Check sheet for the modelled part. Datum: model origin and axes. Units: mm. Round coordinates to 2 decimals unless told otherwise and drop trailing zeros. Write each loop counter-clockwise with the first axis right and the second up, starting at its lowest first coordinate (ties: lowest second). Pieces come first, ordered by that corner, then holes.
from build123d import *

# Parameters (mm, degrees)
SKETCH1_W                = 132
SKETCH1_H                = 150
BOSS_EXTRUDE1_DEPTH      = 5
M6_CLEARANCE_HOLE1_D     = 6.6
M6_CLEARANCE_HOLE1_DEPTH = 10
M6_CLEARANCE_HOLE1_TIP   = 1.982840043
FILLET1_R                = 5


with BuildPart() as part:
    # Sketch1 → Boss-Extrude1 (new body)
    with BuildSketch(Plane(origin=(0, 0, 0), x_dir=(1, 0, 0), z_dir=(0, 1, 0))):
        with Locations((66, 75)):
            Rectangle(SKETCH1_W, SKETCH1_H)
    extrude(amount=BOSS_EXTRUDE1_DEPTH)

    # M6 Clearance Hole1
    with Locations(Plane(origin=(0, 0, 0), x_dir=(-1, 0, 0), z_dir=(0, -1, 0))):
        with Locations((-15, 15), (-117, 15), (-117, 135), (-15, 135)):
            Hole(M6_CLEARANCE_HOLE1_D / 2, depth=M6_CLEARANCE_HOLE1_DEPTH)
            with Locations((0, 0, -(M6_CLEARANCE_HOLE1_DEPTH + M6_CLEARANCE_HOLE1_TIP / 2))):  # 118° drill point
                Cone(0, M6_CLEARANCE_HOLE1_D / 2, M6_CLEARANCE_HOLE1_TIP, mode=Mode.SUBTRACT)

    # Fillet1
    fillet1_edges = [part.edges().sort_by_distance(p)[0] for p in [
        (0, 2.5, -150),
        (132, 2.5, -150),
        (132, 2.5, 0),
        (0, 2.5, 0),
    ]]
    fillet(fillet1_edges, radius=FILLET1_R)


solid = part.part
1. Sectioned sample at A-A, the plane z = -135. Enter the section's corners in (x, y), plus the area to 3 significant figures.
2. Release check for a two-part mould opening along Z. For faces 1 (the cylindrical face through (113.7, 2.5, -15.1)), 2 (the flat face through (65, 5, -76)), 3 (the cylindrical face through (14.28, 2.54, -131.78)), 4 (the cylindrical face through (1, 3, -2)) record: released by +Z, released by -Z, zero draft, split by the parting line, or undercut.
3. Sectioned sample at B-B, the plane x = 15. Enter the section's corners in (y, z).
4. Scan lines: line 1 along Z through (x, y) = (117, 1.1); line 2 along X through (y, z) = (3.8, -15); line 3 along Z through (x, y) = (13.5, 3.05). Record each from-to range of solid material in increasing order.
Computed values:
1. outline: (0, 0) - (11.7, 0) - (11.7, 5) - (0, 5) - close; (18.3, 0) - (113.7, 0) - (113.7, 5) - (18.3, 5) - close; (120.3, 0) - (132, 0) - (132, 5) - (120.3, 5) - close
1. area: 594 mm2
2. face 1: undercut
2. face 2: zero draft
2. face 3: undercut
2. face 4: released by +Z
3. outline: (0, -150) - (5, -150) - (5, -138.3) - (0, -138.3) - close; (0, -131.7) - (5, -131.7) - (5, -18.3) - (0, -18.3) - close; (0, -11.7) - (5, -11.7) - (5, 0) - (0, 0) - close
4. line 1: z = -150 to -138.3, -131.7 to -18.3, -11.7 to 0
4. line 2: x = 0 to 11.7, 18.3 to 113.7, 120.3 to 132
4. line 3: z = -150 to -137.94, -132.06 to -17.94, -12.06 to 0
